Read the model definition and answer for the solid it produces. Units are mm, in the model's axes. A direction names the side the tool comes from. Coordinates: 2 decimals unless noted, no trailing zeros. Write each loop counter-clockwise with the first axis right and the second up, starting at its lowest first coordinate (ties: lowest second). Pieces come first, ordered by that corner, then holes.
from build123d import *

# Parameters (mm, degrees)
PAD_DEPTH = 2.54


with BuildPart() as part:
    # Sketch → Revolution (revolve)
    with BuildSketch(Plane.XZ):
        with BuildLine():
            Line((0, 0), (1.435, 0))
            Line((1.435, 0), (1.435, -1.27))
            Line((1.22, -1.27), (1.435, -1.27))
            Line((1.22, -1.27), (1.22, -3.33))
            Line((0.785, -3.33), (1.22, -3.33))
            Line((0.785, -3.33), (0.785, -7.32302))
            ThreePointArc((0, -8.11), (0.555199, -7.878799), (0.785, -7.32302))
            Line((0, 0), (0, -8.11))
        make_face()
    revolve(axis=Axis((0, 0, 0), (0, 0, 1)))

    # Sketch001 (on Face1 of Revolution) → Pad (new body)
    with BuildSketch(Plane(origin=(0, 0, 0), x_dir=(-1, 0, 0), z_dir=(0, 0, 1))):
        Polygon((0.425, 0.736122), (-0.425, 0.736122), (-0.85, 0), (-0.425, -0.736122), (0.425, -0.736122), (0.85, 0), align=None)
    extrude(amount=PAD_DEPTH)


solid = part.part
Item 1: The part is cut by section D-D (z = -3.75). Give the vertices of the cut face in (x, y) (3 decimals), and give its area (3 significant figures).
Item 2: For faces 1 (the flat face through (1, 0, 0)), 2 (the cylindrical face through (0.749, 0.236, -5.354)), 3 (the flat face through (0, -0.736, 1)), determine the directions among +Z, -Z, +X, -X, +Y, -Y from which every point of the face is accessible in a straight line to the end or side of a thin tool.
Item 3: The part is cut by section B-B (z = 1.75). Give the vertices of the cut face in (x, y) (3 decimals).
Item 4: Given pin 1 (0.9 mm diameter, centred on x = 0, z = 1.5, fed in from +Y); pin 2 (1 mm diameter, centred on x = -1, z = -4, fed in from -Y), each flat-ended and moving along its own axis, determine where each tip first touches the part or whether it passes through.
Item 5: The part is cut by section A-A (x = -1). Give the vertices of the cut face in (y, z), and give its area (3 significant figures).
Item 6: Find the intervals of material crossed by probe 1 along Z at (x, y) = (0.25, 0.95); probe 2 along Y at (x, z) = (0.35, 1.5); probe 3 along Z at (x, y) = (-0.6, 1.25), in increasing order.
Item 7: The part is cut by section C-C (y = -0.9). Give the vertices of the cut face in (x, z), and give its area (3 significant figures).
Answer:
1. outline: circle Ø1.57 at (0, 0)
1. area: 1.94 mm2
2. face 1: +Z
2. face 2: -Z
2. face 3: +Z, +X, -X, -Y
3. outline: (-0.85, 0) - (-0.425, -0.736) - (0.425, -0.736) - (0.85, 0) - (0.425, 0.736) - (-0.425, 0.736) - close
4. pin 1: stops at y = 0.74
4. pin 2: stops at y = -0.61
5. outline: (-1.03, -1.27) - (-0.7, -1.27) - (-0.7, -3.33) - (0.7, -3.33) - (0.7, -1.27) - (1.03, -1.27) - (1.03, 0) - (-1.03, 0) - close
5. area: 5.49 mm2
6. probe 1: z = -3.33 to 0
6. probe 2: y = -0.74 to 0.74
6. probe 3: z = -1.27 to 0
7. outline: (-1.12, -1.27) - (-0.82, -1.27) - (-0.82, -3.33) - (0.82, -3.33) - (0.82, -1.27) - (1.12, -1.27) - (1.12, 0) - (-1.12, 0) - close
7. area: 6.23 mm2
